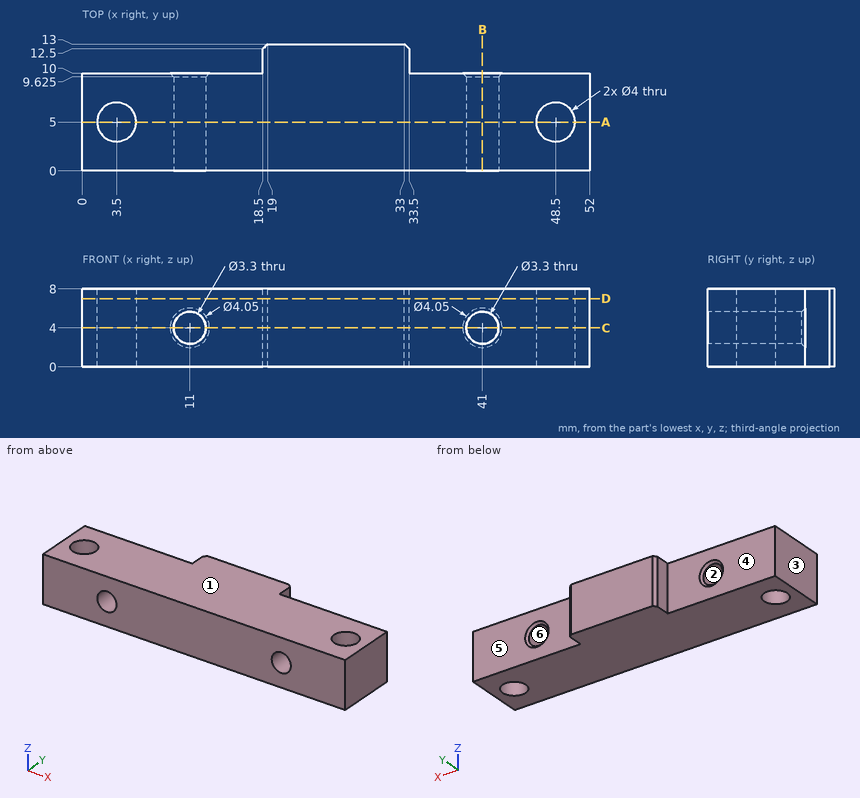
Here's the drawing with two shaded views (mm, measured from the low corner). I have some questions. A direction names the side the tool comes from. Give positions to 0.01 mm unless a question says otherwise; leave off trailing zeros. Loops run counter-clockwise (first coordinate to the right, second up) from the corner with the lowest first, then second, coordinate; pieces in that order, holes last. Notation, with made-up numbers: M 73,-5.5 L 77,-5.5 A22 ccw 77,3.5 Z; hole C -2.5,-5 d3. An arc over 180 degrees is marked long. Use one line per item in the form item = value. Start each with the question number.
(1) I want a section at B-B, the plane x = 41. Write out the boundary of the cut face in (y, z) (3 decimals), and give its area (3 significant figures).
(2) Thinking about a two-plate mould opening in X: for the marked faces 1, 2 and 3, which applies, released by +X, released by -X, zero draft, split by the parting line, or undercut?
(3) On a 3-axis mill with a long thin cutter (end or side, diameter ignored), from which of +Z, -Z, +X, -X, +Y, -Y can I reach the whole of each face in a straight line? I mean the marked faces 4, 5 and 6. Say none if no direction works.
(4) I'm going to push flat-ended pins straight in: P1, Ø4, axis at x = 45.5, z = 7, coming from the +Y side; P2, Ø3, axis at x = 11, z = 4, coming from the -Y side. Where does each tip first touch, or does it pass through?
(5) I want a section at C-C, the plane z = 4. Write out the boundary of the cut face in (x, y) (3 decimals), and give its area (3 significant figures).
(6) I want a section at D-D, the plane z = 7. Write out the boundary of the cut face in (x, y), and give its area (3 significant figures).
(7) Please list where these lines run through material, in increasing order: line 1 (Z direction, x = 41, y = 2.5); line 2 (X direction, y = 2, z = 5.5); line 3 (X direction, y = 7.25, z = 4.25).
(8) I want a section at A-A, the plane y = 5. Write out the boundary of the cut face in (x, z), and give its area (3 significant figures).
Worked out:
q1.outline = M 0,0 L 10,0 L 10,1.975 L 9.625,2.35 L 0,2.35 Z; M 0,5.65 L 9.625,5.65 L 10,6.025 L 10,8 L 0,8 Z
q1.area = 46.9 mm²
q2.face_1 = zero draft
q2.face_2 = undercut
q2.face_3 = released by -X
q3.face_4 = +Z, -Z, -X, +Y
q3.face_5 = +Z, -Z, +X, +Y
q3.face_6 = +Y, -Y
q4.P1 = 10
q4.P2 = through
q5.outline = M 0,0 L 9.35,0 L 9.35,9.625 L 8.975,10 L 0,10 Z; M 12.65,0 L 39.35,0 L 39.35,9.625 L 38.975,10 L 33.5,10 L 33.5,12.5 L 33,13 L 19,13 L 18.5,12.5 L 18.5,10 L 13.025,10 L 12.65,9.625 Z; M 42.65,0 L 52,0 L 52,10 L 43.025,10 L 42.65,9.625 Z; hole C 3.5,5 d4; hole C 48.5,5 d4
q5.area = 473 mm²
q6.outline = M 0,0 L 52,0 L 52,10 L 33.5,10 L 33.5,12.5 L 33,13 L 19,13 L 18.5,12.5 L 18.5,10 L 0,10 Z; hole C 3.5,5 d4; hole C 48.5,5 d4
q6.area = 540 mm²
q7.line_1 = 0 to 2.35, 5.65 to 8
q7.line_2 = 0 to 10.31, 11.69 to 40.31, 41.69 to 52
q7.line_3 = 0 to 9.37, 12.63 to 39.37, 42.63 to 52
q8.outline = M 0,0 L 1.5,0 L 1.5,8 L 0,8 Z; M 5.5,0 L 46.5,0 L 46.5,8 L 5.5,8 Z; M 50.5,0 L 52,0 L 52,8 L 50.5,8 Z; hole C 11,4 d3.3; hole C 41,4 d3.3
q8.area = 335 mm²
